Geometry check sheet. Reference: the model listing, model coordinates, mm. A direction names the side the tool comes from. Coordinates: 2 decimals unless noted, no trailing zeros. Order: outer loops, then holes, each group sorted by start corner. A loop starts at its lowest first (then second) coordinate and runs counter-clockwise, first axis right, second up. Notation, with made-up numbers: (37, 27.5) - (90, 27.5) arc R34 ccw to (90, 62.5) - close; hole circle Ø5 at (68, 82). An arc over 180 degrees is marked (long way). Use CSV: the item, a comma, the result in double quotes. Start each with the question number.
1) Draft check along X on faces 6 (the cylindrical face through (-0.78, 13.4, 1.97)), 7 (the flat face through (22, 4, 2)). Enter one of: released by +X, released by -X, zero draft, split by the parting line, or undercut.
2) Depth check by flat-ended pin: P1, Ø2.5, axis at x = 4.5, y = 0, coming from the +Z side; P2, Ø2, axis at x = 20, z = 2.5, coming from the -Y side; P3, Ø1, axis at y = 0.5, z = 0.5, coming from the +X side; P4, Ø2, axis at y = 2.5, z = 0.5, coming from the +X side. Enter the tip coordinate at first touch or a pass-through.
3) Thickness scan on probe 1 along X at (y, z) = (11.75, 1.95); probe 2 along X at (y, z) = (1, 1.95); probe 3 along Y at (x, z) = (22, 3.8). Record the ranges inside material, lowest first. Write a range as [from, to].
4) Sectioned sample at A-A, the plane x = 27. Record the cut outline in (y, z), and give its area (3 significant figures).
5) Tool access check on faces 1 (the cylindrical face through (8.6, 10.3, 2)), 2 (the cylindrical face through (-0.641, -12.073, 1.972)), 3 (the cylindrical face through (-10.94, 5.15, 1.97)), 4 (the flat face through (21, -4, 2)), 5 (the flat face through (4.2, 1.5, 0)). Record the directions out of +Z, -Z, +X, -X, +Y, -Y that give a thin tool (end or side, any length) a straight path to the whole face; none if there is none.
6) Sectioned sample at C-C, the plane y = -9. Record the cut outline in (x, z).
7) Sectioned sample at B-B, the plane z = 3.25. Count the separate pieces of the cut face and the enclosed holes in it, and give its area (3 significant figures).
from build123d import *

# Parameters (mm, degrees)
SKETCH1_R           = 1.75
BOSS_EXTRUDE1_DEPTH = 4
SKETCH2_R           = 1.3
SKETCH2_R_2         = 2.4
CUT_EXTRUDE1_DEPTH  = 20


with BuildPart() as part:
    # Sketch1 → Boss-Extrude1 (new body)
    with BuildSketch(Plane.XY):
        with BuildLine():
            ThreePointArc((13.776114953, 4), (13.893050478, 4.110818553), (14.006628151, 4.225076075))
            ThreePointArc((14.006628151, 4.225076075), (13.913956833, 4.520918628), (13.815037615, 4.814731115))
            ThreePointArc((13.815037615, 4.814731115), (12.481386111, 4.882828881), (11.171803009, 4.621570895))
            ThreePointArc((11.171803009, 4.621570895), (10.939359064, 5.147671635), (10.682156823, 5.662122005))
            ThreePointArc((10.682156823, 5.662122005), (11.718219248, 6.50464102), (12.515850479, 7.575644315))
            ThreePointArc((12.515850479, 7.575644315), (12.35251755, 7.839146011), (12.183637866, 8.099127629))
            ThreePointArc((12.183637866, 8.099127629), (10.874950252, 7.833420336), (9.671482329, 7.254690176))
            ThreePointArc((9.671482329, 7.254690176), (9.315505105, 7.706456036), (8.938444741, 8.140780406))
            ThreePointArc((8.938444741, 8.140780406), (9.7324314, 9.214488384), (10.238655891, 10.450206961))
            ThreePointArc((10.238655891, 10.450206961), (10.01492416, 10.664811019), (9.786695342, 10.874626167))
            ThreePointArc((9.786695342, 10.874626167), (8.585201272, 10.291809183), (7.563466846, 9.431970593))
            ThreePointArc((7.563466846, 9.431970593), (7.1063237, 9.781015462), (6.633097302, 10.107923633))
            ThreePointArc((6.633097302, 10.107923633), (7.135119095, 11.345355554), (7.318128899, 12.668144672))
            ThreePointArc((7.318128899, 12.668144672), (7.048056252, 12.820366729), (6.774818757, 12.966831949))
            ThreePointArc((6.774818757, 12.966831949), (5.756012523, 12.103525808), (4.980210924, 11.016605609))
            ThreePointArc((4.980210924, 11.016605609), (4.450625842, 11.240997714), (3.910967965, 11.439948845))
            ThreePointArc((3.910967965, 11.439948845), (4.089481015, 12.763352309), (3.937776954, 14.090096262))
            ThreePointArc((3.937776954, 14.090096262), (3.638333049, 14.170371647), (3.337255394, 14.244283992))
            ThreePointArc((3.337255394, 14.244283992), (2.565152337, 13.154733392), (2.084030034, 11.909026779))
            ThreePointArc((2.084030034, 11.909026779), (1.515278794, 11.994666739), (0.943098128, 12.053159997))
            ThreePointArc((0.943098128, 12.053159997), (0.786885803, 13.379380698), (0.31, 14.626715284))
            ThreePointArc((0.31, 14.626715284), (0, 14.63), (-0.31, 14.626715284))
            ThreePointArc((-0.31, 14.626715284), (-0.786885803, 13.379380698), (-0.943098128, 12.053159997))
            ThreePointArc((-0.943098128, 12.053159997), (-1.515278794, 11.994666739), (-2.084030034, 11.909026779))
            ThreePointArc((-2.084030034, 11.909026779), (-2.565152337, 13.154733392), (-3.337255394, 14.244283992))
            ThreePointArc((-3.337255394, 14.244283992), (-3.638333049, 14.170371647), (-3.937776954, 14.090096262))
            ThreePointArc((-3.937776954, 14.090096262), (-4.089481015, 12.763352309), (-3.910967965, 11.439948845))
            ThreePointArc((-3.910967965, 11.439948845), (-4.450625842, 11.240997714), (-4.980210924, 11.016605609))
            ThreePointArc((-4.980210924, 11.016605609), (-5.756012523, 12.103525808), (-6.774818757, 12.966831949))
            ThreePointArc((-6.774818757, 12.966831949), (-7.048056252, 12.820366729), (-7.318128899, 12.668144672))
            ThreePointArc((-7.318128899, 12.668144672), (-7.135119095, 11.345355554), (-6.633097302, 10.107923633))
            ThreePointArc((-6.633097302, 10.107923633), (-7.1063237, 9.781015462), (-7.563466846, 9.431970593))
            ThreePointArc((-7.563466846, 9.431970593), (-8.585201272, 10.291809183), (-9.786695342, 10.874626167))
            ThreePointArc((-9.786695342, 10.874626167), (-10.01492416, 10.664811019), (-10.238655891, 10.450206961))
            ThreePointArc((-10.238655891, 10.450206961), (-9.7324314, 9.214488384), (-8.938444741, 8.140780406))
            ThreePointArc((-8.938444741, 8.140780406), (-9.315505105, 7.706456036), (-9.671482329, 7.254690176))
            ThreePointArc((-9.671482329, 7.254690176), (-10.874950252, 7.833420336), (-12.183637866, 8.099127629))
            ThreePointArc((-12.183637866, 8.099127629), (-12.35251755, 7.839146011), (-12.515850479, 7.575644315))
            ThreePointArc((-12.515850479, 7.575644315), (-11.718219248, 6.50464102), (-10.682156823, 5.662122005))
            ThreePointArc((-10.682156823, 5.662122005), (-10.939359064, 5.147671635), (-11.171803009, 4.621570895))
            ThreePointArc((-11.171803009, 4.621570895), (-12.481386111, 4.882828881), (-13.815037615, 4.814731115))
            ThreePointArc((-13.815037615, 4.814731115), (-13.913956833, 4.520918628), (-14.006628151, 4.225076075))
            ThreePointArc((-14.006628151, 4.225076075), (-12.967708283, 3.386083139), (-11.754669706, 2.827691655))
            ThreePointArc((-11.754669706, 2.827691655), (-11.875852861, 2.265440093), (-11.970158218, 1.698061317))
            ThreePointArc((-11.970158218, 1.698061317), (-13.303570578, 1.625431329), (-14.578387742, 1.227807338))
            ThreePointArc((-14.578387742, 1.227807338), (-14.601131037, 0.918625301), (-14.617317864, 0.609030766))
            ThreePointArc((-14.617317864, 0.609030766), (-13.402388515, 0.054765201), (-12.088593461, -0.184412961))
            ThreePointArc((-12.088593461, -0.184412961), (-12.066143147, -0.759137381), (-12.016384363, -1.332143698))
            ThreePointArc((-12.016384363, -1.332143698), (-13.289842779, -1.734098051), (-14.425724151, -2.43626409))
            ThreePointArc((-14.425724151, -2.43626409), (-14.370862478, -2.741388632), (-14.309547736, -3.045282186))
            ThreePointArc((-14.309547736, -3.045282186), (-12.994947386, -3.279993836), (-11.662946429, -3.184930232))
            ThreePointArc((-11.662946429, -3.184930232), (-0.426838607, -12.082462862), (11.409123542, -4))
            Line((11.409123542, -4), (30.75, -4))
            ThreePointArc((30.75, -4), (34.75, 0), (30.75, 4))
            Line((30.75, 4), (13.776114953, 4))
        make_face()
        Circle(SKETCH1_R, mode=Mode.SUBTRACT)
        with Locations((30.75, 0)):
            Circle(SKETCH1_R, mode=Mode.SUBTRACT)
    extrude(amount=BOSS_EXTRUDE1_DEPTH)

    # Sketch2 → Cut-Extrude1 (cut)
    with BuildSketch(Plane.XY.offset(4)):
        with Locations((4.5, 0)):
            Circle(SKETCH2_R)
        with Locations((-4.5, 0)):
            Circle(SKETCH2_R)
        Circle(SKETCH2_R_2)
    extrude(amount=-CUT_EXTRUDE1_DEPTH, mode=Mode.SUBTRACT)


solid = part.part
Evaluation:
1,face 6,"undercut"
1,face 7,"zero draft"
2,P1,"through"
2,P2,"y = -4"
2,P3,"x = 34.75"
2,P4,"x = 34.46"
3,probe 1,"[-7.23, -5.46], [-3.98, 3.98], [5.46, 7.23]"
3,probe 2,"[-14.6, -5.33], [-3.67, -2.18], [2.18, 3.67], [5.33, 29.31], [32.19, 34.62]"
3,probe 3,"[-4, 4]"
4,outline,"(-4, 0) - (4, 0) - (4, 4) - (-4, 4) - close"
4,area,"32.0 mm²"
5,face 1,"+Z, -Z, +Y"
5,face 2,"+Z, -Z, -Y"
5,face 3,"+Z, -Z"
5,face 4,"+Z, -Z, +X, -Y"
5,face 5,"-Z, +X, -X, +Y, -Y"
6,outline,"(-8.07, 0) - (8.07, 0) - (8.07, 4) - (-8.07, 4) - close"
7,separate pieces,"1"
7,enclosed holes,"4"
7,area,"644 mm²"
